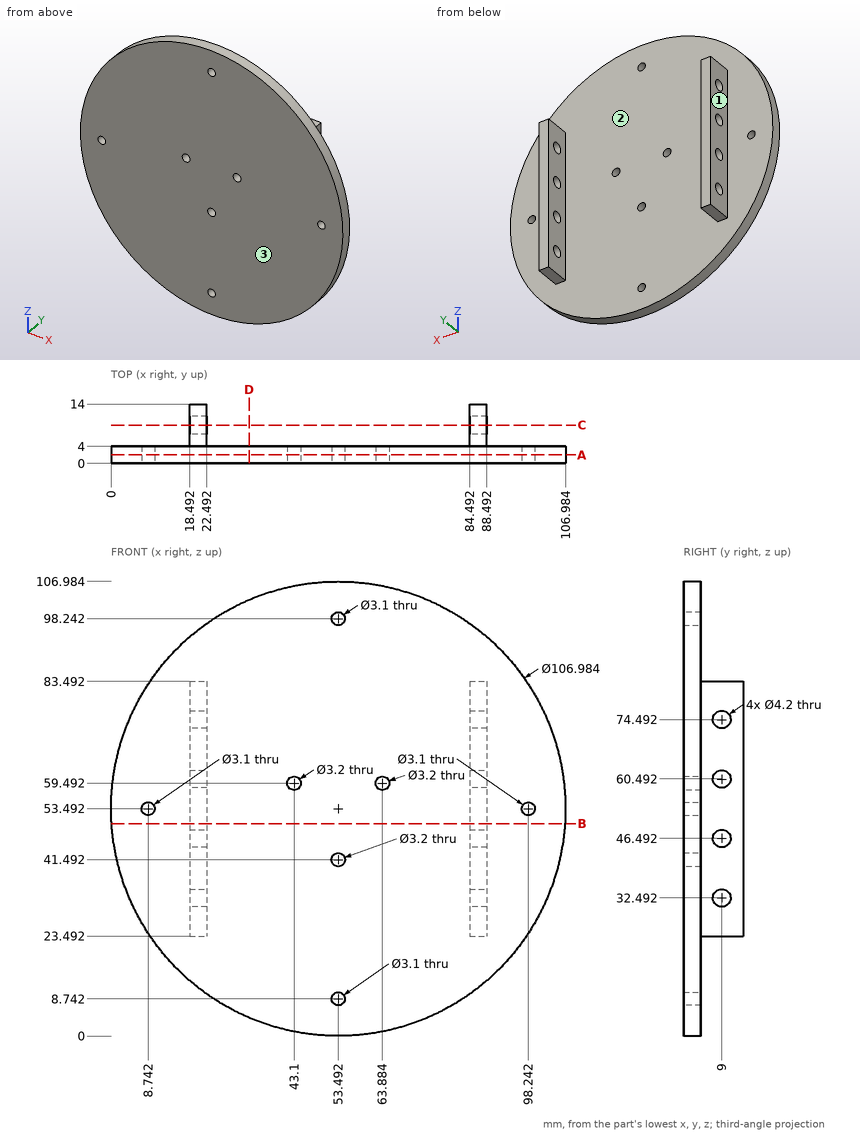
Geometry: see drawing. Coordinates: mm, zero at the bounding-box minimum. Give positions to 0.01 mm unless a question says otherwise; leave off trailing zeros. Loops run counter-clockwise (first coordinate to the right, second up) from the corner with the lowest first, then second, coordinate; pieces in that order, holes last. Notation, with made-up numbers: M 4,18 L 22,18 A36 cw 22,54 Z; hole C 24,50.5 d1. An arc over 180 degrees is marked long. Answer as CSV lines item,"result". Start each with the question number.
1. Section A-A on y = 2. Return loops of the section in (x, z), plus the area to 4 significant figures.
2. Line query: L1, parallel to X at y = 6.25, z = 28.5; L2, parallel to Z at x = 86, y = 8.5; L3, parallel to Y at x = 64, z = 43.5. Output: solid intervals per line, ascending.
3. Section D-D on x = 32.5. Return loops of the section in (y, z).
4. Pin query (flat end, axial travel): P1, Ø3.5, axis at x = 53.49, z = 41.49, coming from the +Y side; P2, Ø4.5, axis at x = 19.5, y = 9.5, coming from the +Z side; P3, Ø10, axis at x = 88.5, z = 37, coming from the -Y side; P4, Ø5, axis at y = 9, z = 60.49, coming from the -X side. Return the tip coordinate at first contact, or that it passes through.
5. Section B-B on z = 50. Return loops of the section in (x, y), plus the area to 3 significant figures.
6. Section C-C on y = 9. State how many separate pieces and enclosed holes the cut face has.
7. Pull-direction query (X, two-part tool) for the marked faces 1, 2 and 3; classes: released by +X, released by -X, zero draft, split by the parting line, or undercut.
Computed values:
1,outline,"C 53.49,53.49 d106.98; hole C 8.74,53.49 d3.1; hole C 43.1,59.49 d3.2; hole C 53.49,41.49 d3.2; hole C 53.49,8.74 d3.1; hole C 53.49,98.24 d3.1; hole C 63.88,59.49 d3.2; hole C 98.24,53.49 d3.1"
1,area,"8,935 mm²"
2,L1,"x = 18.49 to 22.49, 84.49 to 88.49"
2,L2,"z = 23.49 to 30.45, 34.53 to 44.45, 48.53 to 58.45, 62.53 to 72.45, 76.53 to 83.49"
2,L3,"y = 0 to 4"
3,outline,"M 0,4.29 L 4,4.29 L 4,102.69 L 0,102.69 Z"
4,P1,"stops at y = 4"
4,P2,"stops at z = 83.49"
4,P3,"stops at y = 0"
4,P4,"stops at x = 18.49"
5,outline,"M 0.11,0 L 106.87,0 L 106.87,4 L 88.49,4 L 88.49,14 L 84.49,14 L 84.49,4 L 22.49,4 L 22.49,14 L 18.49,14 L 18.49,4 L 0.11,4 Z"
5,area,"507 mm²"
6,separate pieces,"10"
6,enclosed holes,"0"
7,face 1,"released by -X"
7,face 2,"undercut"
7,face 3,"zero draft"
